The model under review builds one solid part; all positions refer to its coordinate system, in mm. Coordinates: 2 decimals unless noted, no trailing zeros. Write each loop counter-clockwise with the first axis right and the second up, starting at its lowest first coordinate (ties: lowest second). Pieces come first, ordered by that corner, then holes.
```python
from build123d import *

# Parameters (mm, degrees)
SKETCH1_W           = 125
SKETCH1_H           = 239.7125
BOSS_EXTRUDE1_DEPTH = 5
CUT_EXTRUDE1_REACH  = 272.392
SKETCH2_R           = 5


with BuildPart() as part:
    # Sketch1 → Boss-Extrude1 (new body)
    with BuildSketch(Plane(origin=(0, 0, 0), x_dir=(1, 0, 0), z_dir=(0, 1, 0))):
        with Locations((62.5, -119.85625)):
            Rectangle(SKETCH1_W, SKETCH1_H)
    extrude(amount=BOSS_EXTRUDE1_DEPTH)

    # Sketch2 → Cut-Extrude1 (cut, up to next)
    with BuildSketch(Plane.XZ, mode=Mode.PRIVATE) as cut_extrude1_sk1:
        with Locations(Location((12.5, 229.7125, 0), (0, 0, 270))):
            Circle(SKETCH2_R)
    cut_extrude1_tool1 = extrude(cut_extrude1_sk1.sketch, amount=-CUT_EXTRUDE1_REACH, mode=Mode.PRIVATE) & part.part
    # Sketch2 → Cut-Extrude1 (cut, up to next)
    with BuildSketch(Plane.XZ, mode=Mode.PRIVATE) as cut_extrude1_sk2:
        with Locations(Location((112.5, 229.7125, 0), (0, 0, 270))):
            Circle(SKETCH2_R)
    cut_extrude1_tool2 = extrude(cut_extrude1_sk2.sketch, amount=-CUT_EXTRUDE1_REACH, mode=Mode.PRIVATE) & part.part
    # Sketch2 → Cut-Extrude1 (cut, up to next)
    with BuildSketch(Plane.XZ, mode=Mode.PRIVATE) as cut_extrude1_sk3:
        with Locations(Location((12.5, 10, 0), (0, 0, 270))):
            Circle(SKETCH2_R)
    cut_extrude1_tool3 = extrude(cut_extrude1_sk3.sketch, amount=-CUT_EXTRUDE1_REACH, mode=Mode.PRIVATE) & part.part
    # Sketch2 → Cut-Extrude1 (cut, up to next)
    with BuildSketch(Plane.XZ, mode=Mode.PRIVATE) as cut_extrude1_sk4:
        with Locations(Location((112.5, 10, 0), (0, 0, 270))):
            Circle(SKETCH2_R)
    cut_extrude1_tool4 = extrude(cut_extrude1_sk4.sketch, amount=-CUT_EXTRUDE1_REACH, mode=Mode.PRIVATE) & part.part
    add(cut_extrude1_tool1.solids().sort_by_distance((12.5, 0, 229.7125))[0], mode=Mode.SUBTRACT)
    add(cut_extrude1_tool2.solids().sort_by_distance((112.5, 0, 229.7125))[0], mode=Mode.SUBTRACT)
    add(cut_extrude1_tool3.solids().sort_by_distance((12.5, 0, 10))[0], mode=Mode.SUBTRACT)
    add(cut_extrude1_tool4.solids().sort_by_distance((112.5, 0, 10))[0], mode=Mode.SUBTRACT)


solid = part.part
```
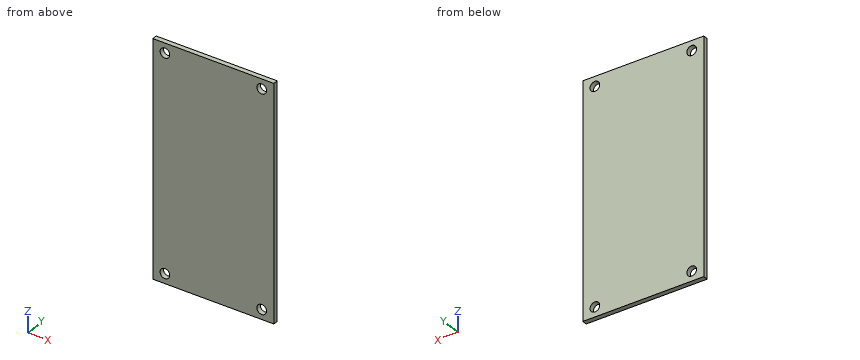
Item 1: To check wall thickness, follow line 1 along X through (y, z) = (1.55, 10); line 2 along Z through (x, y) = (110, 3.15). State the ranges of each line that lie inside material, in increasing order.
Solved:
line 1: x = 0 to 7.5, 17.5 to 107.5, 117.5 to 125
line 2: z = 0 to 5.67, 14.33 to 225.38, 234.04 to 239.71
Item 2: Take a section at B-B, the plane x = 112.5. Write out the cut boundary in (y, z), plus the area to 3 significant figures.
Solved:
outline: (0, 0) - (5, 0) - (5, 5) - (0, 5) - close; (0, 15) - (5, 15) - (5, 224.71) - (0, 224.71) - close; (0, 234.71) - (5, 234.71) - (5, 239.71) - (0, 239.71) - close
area: 1,100 mm2
Item 3: Take a section at A-A, the plane z = 10. Write out the cut boundary in (x, y).
Solved:
outline: (0, 0) - (7.5, 0) - (7.5, 5) - (0, 5) - close; (17.5, 0) - (107.5, 0) - (107.5, 5) - (17.5, 5) - close; (117.5, 0) - (125, 0) - (125, 5) - (117.5, 5) - close
Item 4: For pin 1 (8 mm diameter, centred on x = 12.5, z = 229.71, fed in from +Y), flat-tipped, find the tip position at first contact; note if it passes through.
Solved:
pin 1: passes through
